Geometry: see drawing. Coordinates: mm, zero at the bounding-box minimum. A direction names the side the tool comes from. Give positions to 0.01 mm unless a question says otherwise; leave off trailing zeros. Loops run counter-clockwise (first coordinate to the right, second up) from the corner with the lowest first, then second, coordinate; pieces in that order, holes last. Notation, with made-up numbers: M -31,-16 L -22,-16 A34 ccw -22,18 Z; hole C -22,41.25 d7. An arc over 180 degrees is marked long. Use CSV: the item, a comma, the result in double quotes. Start each with the question number.
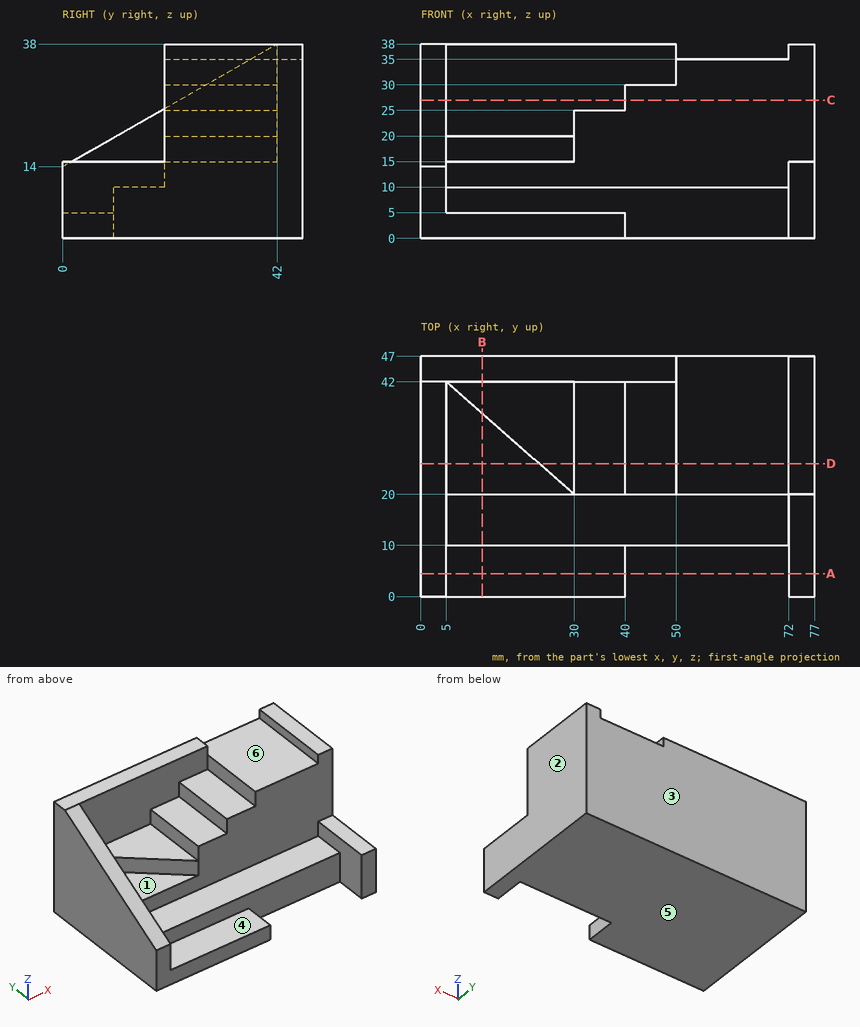
Item 1: Set-up query: the marked faces 4, 5 and 6. Return all of +Z, -Z, +X, -X, +Y, -Y with unobstructed straight access to the full face (end or side cutting, diameter ignored); none if empty.
Item 2: First-contact query: pin 1 Ø3 at (x, y) = (43, 28) entering from +Z; pin 2 Ø3 at (x, z) = (43, 5.5) entering from -Y; pin 3 Ø11 at (x, y) = (49.5, 14) entering from +Z. Flat tips, straight axial feed; report the tip coordinate or a pass-through.
Item 3: Material intervals for line 1 (X direction, y = 24, z = 22.5); line 2 (X direction, y = 38.5, z = 35.5); line 3 (Z direction, x = 16, y = 14.5), sorted ascending.
Item 4: Section C-C (z = 27). Output: boundary loops of the cut face in (x, y), then the cut area to 3 significant figures.
Item 5: Section A-A (y = 4.5). Output: boundary loops of the cut face in (x, z).
Item 6: Mould query, pull axis X, two halves, no side actions, for the marked faces 1, 2 and 3. Classes: +X half, -X half, draft (parallel to the pull), parting line (faces both ways), or undercut.
Item 7: Section D-D (y = 26). Output: boundary loops of the cut face in (x, z).
Item 8: Section B-B (x = 12). Output: boundary loops of the cut face in (y, z).
Recorded:
1,face 4,"+Z, -Y"
1,face 5,"-Z, +X, -X, +Y, -Y"
1,face 6,"+Z, +Y, -Y"
2,pin 1,"z = 30"
2,pin 2,"y = 10"
2,pin 3,"z = 10"
3,line 1,"0 to 5, 30 to 77"
3,line 2,"0 to 5, 72 to 77"
3,line 3,"0 to 10"
4,outline,"M 0,22.75 L 5,22.75 L 5,42 L 40,42 L 40,20 L 77,20 L 77,47 L 0,47 Z"
4,area,"1,300 mm²"
5,outline,"M 0,0 L 40,0 L 40,5 L 5,5 L 5,16.57 L 0,16.57 Z; M 72,0 L 77,0 L 77,15 L 72,15 Z"
6,face 1,"undercut"
6,face 2,"+X half"
6,face 3,"draft"
7,outline,"M 0,0 L 77,0 L 77,38 L 72,38 L 72,35 L 50,35 L 50,30 L 40,30 L 40,25 L 30,25 L 30,20 L 23.18,20 L 23.18,15 L 5,15 L 5,28.86 L 0,28.86 Z"
8,outline,"M 0,0 L 47,0 L 47,38 L 42,38 L 42,20 L 35.84,20 L 35.84,15 L 20,15 L 20,10 L 10,10 L 10,5 L 0,5 Z"
